Can you work these out from the drawing? Everything is in mm from the part's minimum corner. A direction names the side the tool comes from. Round coordinates to 2 decimals unless told otherwise and drop trailing zeros. Order: outer loops, then holes, each group sorted by start corner. A loop starts at its lowest first (then second) coordinate and runs counter-clockwise, first axis right, second up. Notation, with made-up numbers: (80.25, 53) -> (102.25, 53) arc R35 cw to (102.25, 87) -> close; hole circle Ø8 at (89.25, -14). An arc over 180 degrees is marked (long way). One line per item, written item: value.
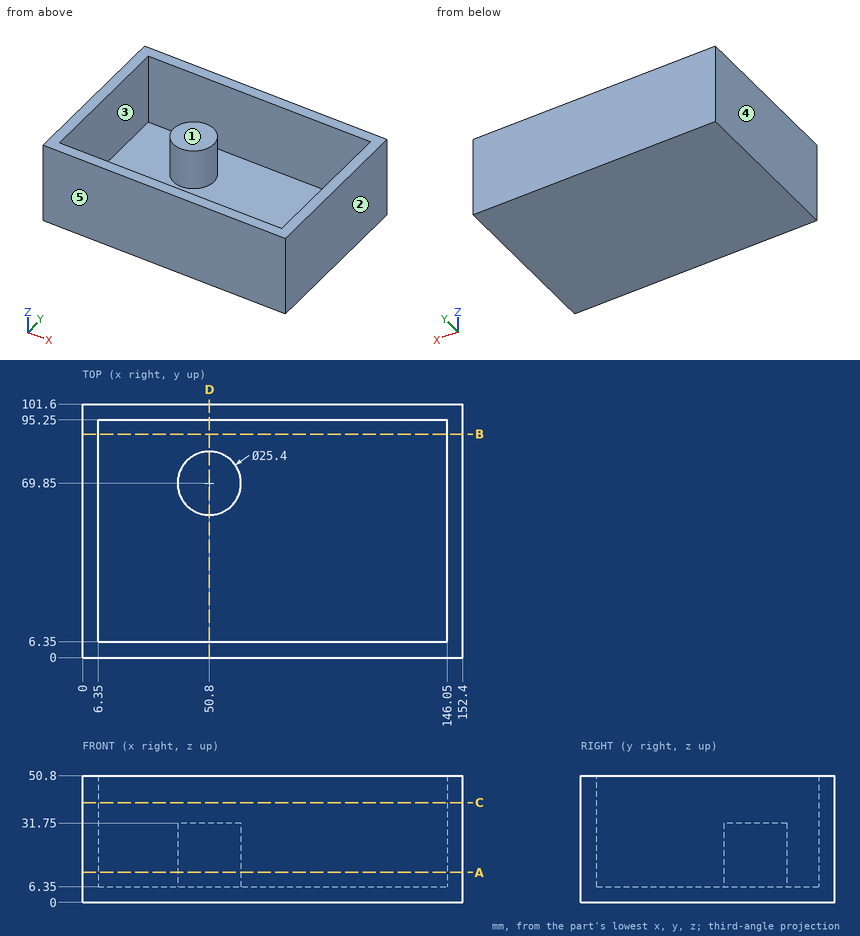
Q1. I want a section at C-C on z = 40. Write out the boundary of the cut face in (x, y), then the cut area to 3 significant figures.
Answers:
outline: (0, 0) -> (152.4, 0) -> (152.4, 101.6) -> (0, 101.6) -> close; hole (6.35, 6.35) -> (146.05, 6.35) -> (146.05, 95.25) -> (6.35, 95.25) -> close
area: 3,060 mm2
Q2. I want a section at A-A on z = 12. Write out the boundary of the cut face in (x, y).
Answers:
outline: (0, 0) -> (152.4, 0) -> (152.4, 101.6) -> (0, 101.6) -> close; circle Ø25.4 at (50.8, 69.85); hole (6.35, 6.35) -> (146.05, 6.35) -> (146.05, 95.25) -> (6.35, 95.25) -> close
Q3. If we mould it in two halves opening along Y, with no side actions, what happens to the marked faces 3, 4 and 5? For each: pulls with the +Y half, pulls with the -Y half, needs draft (parallel to the pull), parting line crosses it, or undercut.
Answers:
face 3: undercut
face 4: needs draft
face 5: pulls with the -Y half
Q4. I want a section at B-B on y = 89.5. Write out the boundary of the cut face in (x, z).
Answers:
outline: (0, 0) -> (152.4, 0) -> (152.4, 50.8) -> (146.05, 50.8) -> (146.05, 6.35) -> (6.35, 6.35) -> (6.35, 50.8) -> (0, 50.8) -> close
Q5. For P1, Ø8, axis at x = 27.5, y = 54, coming from the +Z side, with a flat end and sliding along its axis, tell me the tip position at first contact or that it passes through.
Answers:
P1: z = 6.35
Q6. Which directions (+Z, -Z, +X, -X, +Y, -Y) give clear straight access to the entire face, cutting with the end or side of a thin tool? Please do the marked faces 1 and 2.
Answers:
face 1: +Z
face 2: +Z, -Z, +X, +Y, -Y
Q7. I want a section at D-D on x = 50.8. Write out the boundary of the cut face in (y, z).
Answers:
outline: (0, 0) -> (101.6, 0) -> (101.6, 50.8) -> (95.25, 50.8) -> (95.25, 6.35) -> (82.55, 6.35) -> (82.55, 31.75) -> (57.15, 31.75) -> (57.15, 6.35) -> (6.35, 6.35) -> (6.35, 50.8) -> (0, 50.8) -> close
Q8. I need wall thicknesses on line 1 along X through (y, z) = (56, 31); line 2 along Y through (x, z) = (18, 29); line 3 along Y through (x, z) = (45, 30). Which ranges of each line are inside material? Lowest first, please.
Answers:
line 1: 0 to 6.35, 146.05 to 152.4
line 2: 0 to 6.35, 95.25 to 101.6
line 3: 0 to 6.35, 58.55 to 81.15, 95.25 to 101.6
